Build history of the part. All positions in model axes, mm. Face numbers are marked on the shaded views. A direction names the side the tool comes from. Give positions to 0.01 mm unless a question says otherwise; leave off trailing zeros. Order: outer loops, then holes, each group sorted by start corner. A loop starts at its lowest first (then second) coordinate and runs counter-clockwise, first axis right, second up. Notation, with made-up numbers: (75, 83.25) - (96, 83.25) arc R21 ccw to (96, 122.25) - close; hole circle Ø1 at (43.5, -10.5). An arc over 180 degrees is marked (long way). Use a Markdown table: item, result.
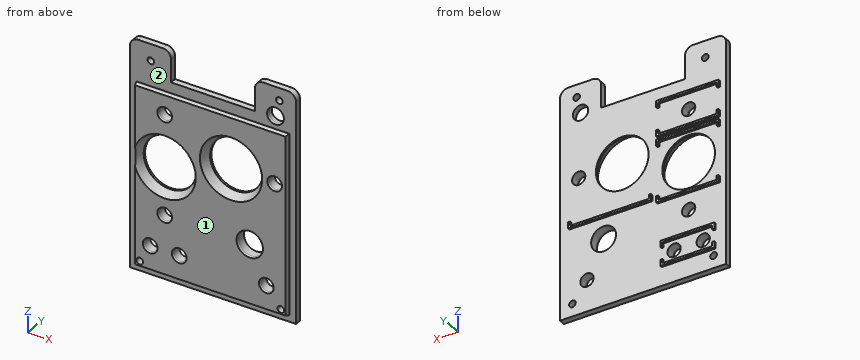
from build123d import *
from OCP.BRepFilletAPI import BRepFilletAPI_MakeChamfer

# Parameters (mm, degrees)
SKETCH1_W           = 80
SKETCH1_H           = 110
BOSS_EXTRUDE1_DEPTH = 3
SKETCH2_W           = 40.4
SKETCH2_H           = 3
CUT_EXTRUDE1_DEPTH  = 15
FILLET1_R           = 4
SKETCH7_W           = 73.6
SKETCH7_H           = 86.6
BOSS_EXTRUDE2_DEPTH = 2
SKETCH3_R           = 12.7
CUT_EXTRUDE2_DEPTH  = 69.190908485
SKETCH4_R           = 6
SKETCH4_R_2         = 3.2
SKETCH4_R_3         = 3.7
SKETCH4_R_4         = 1.6
CUT_EXTRUDE3_DEPTH  = 69.190908485
CHAMFER2_SIZE       = 1.5
CHAMFER2_SIZE2      = 0.545955351
CHAMFER3_SIZE       = 2.309401077
CHAMFER3_SIZE_2     = 4
BOSS_EXTRUDE3_DEPTH = 1
CHAMFER4_SIZE       = 1
CHAMFER4_SIZE2      = 0.363970234


with BuildPart() as part:
    # Sketch1 → Boss-Extrude1 (new body)
    with BuildSketch(Plane(origin=(0, 0, 0), x_dir=(1, 0, 0), z_dir=(0, 1, 0))):
        Rectangle(SKETCH1_W, SKETCH1_H)
    extrude(amount=BOSS_EXTRUDE1_DEPTH)

    # Sketch2 → Cut-Extrude1 (cut)
    with BuildSketch(Plane.XY.offset(55)):
        with Locations((0, 1.5)):
            Rectangle(SKETCH2_W, SKETCH2_H)
    extrude(amount=-CUT_EXTRUDE1_DEPTH, mode=Mode.SUBTRACT)

    # Fillet1
    fillet1_edges = [part.edges().sort_by_distance(p)[0] for p in [
        (-20.2, 1.5, 55),
        (20.2, 1.5, 55),
        (40, 1.5, 55),
        (-40, 1.5, 55),
    ]]
    fillet(fillet1_edges, radius=FILLET1_R)

    # Sketch7 → Boss-Extrude2 (add)
    with BuildSketch(Plane.XZ):
        with Locations((0, -8.5)):
            Rectangle(SKETCH7_W, SKETCH7_H)
    extrude(amount=BOSS_EXTRUDE2_DEPTH)

    # Sketch3 → Cut-Extrude2 (cut, through all)
    with BuildSketch(Plane(origin=(0, 3, 0), x_dir=(1, 0, 0), z_dir=(0, 1, 0))):
        with Locations(Location((-22, 0, 0), (0, 0, 270))):
            Circle(SKETCH3_R)
        with Locations(Location((10, -10, 0), (0, 0, 270))):
            Circle(SKETCH3_R)
    extrude(amount=-CUT_EXTRUDE2_DEPTH, mode=Mode.SUBTRACT)

    # Sketch4 → Cut-Extrude3 (cut, through all)
    with BuildSketch(Plane(origin=(0, 3, 0), x_dir=(1, 0, 0), z_dir=(0, 1, 0))):
        with Locations(Location((19, 23, 0), (0, 0, 270))):
            Circle(SKETCH4_R)
        with Locations(Location((-22, 23, 0), (0, 0, 270))):
            Circle(SKETCH4_R_2)
        with Locations(Location((31, -10, 0), (0, 0, 270))):
            Circle(SKETCH4_R_2)
        with Locations(Location((30.1, -41, 0), (0, 0, 270))):
            Circle(SKETCH4_R_3)
        with Locations(Location((-29, 40, 0), (0, 0, 270))):
            Circle(SKETCH4_R_2)
        with Locations(Location((-15, 40, 0), (0, 0, 270))):
            Circle(SKETCH4_R_2)
        with Locations(Location((27, 40, 0), (0, 0, 270))):
            Circle(SKETCH4_R_2)
        with Locations(Location((-22, -25, 0), (0, 0, 270))):
            Circle(SKETCH4_R_2)
        with Locations(Location((-30, -47, 0), (0, 0, 270))):
            Circle(SKETCH4_R_4)
        with Locations(Location((-34, 49, 0), (0, 0, 270))):
            Circle(SKETCH4_R_4)
        with Locations(Location((34, 49, 0), (0, 0, 270))):
            Circle(SKETCH4_R_4)
        with Locations(Location((32, -49, 0), (0, 0, 270))):
            Circle(SKETCH4_R_4)
    extrude(amount=-CUT_EXTRUDE3_DEPTH, mode=Mode.SUBTRACT)

    # Chamfer2: one chamfer whose edges measure the first distance from different faces: ONE call of the kernel's chamfer builder (chamfer() names one face for all edges)
    chamfer2_edges_1 = [part.edges().sort_by_distance(p)[0] for p in [
        (-36.8, -2, -8.5),
    ]]
    chamfer2_side_1 = [part.faces().sort_by_distance(p)[0] for p in [
        (-36.8, -1, -8.5),
    ]]
    chamfer2_edges_2 = [part.edges().sort_by_distance(p)[0] for p in [
        (0, -2, -51.8),
    ]]
    chamfer2_side_2 = [part.faces().sort_by_distance(p)[0] for p in [
        (0, -1, -51.8),
    ]]
    chamfer2_edges_3 = [part.edges().sort_by_distance(p)[0] for p in [
        (36.8, -2, -8.5),
    ]]
    chamfer2_side_3 = [part.faces().sort_by_distance(p)[0] for p in [
        (36.8, -1, -8.5),
    ]]
    chamfer2_edges_4 = [part.edges().sort_by_distance(p)[0] for p in [
        (0, -2, 34.8),
    ]]
    chamfer2_side_4 = [part.faces().sort_by_distance(p)[0] for p in [
        (0, -1, 34.8),
    ]]
    chamfer2 = BRepFilletAPI_MakeChamfer(part.part.solid().wrapped)
    for e in chamfer2_edges_1:
        chamfer2.Add(CHAMFER2_SIZE, CHAMFER2_SIZE2, e.wrapped, chamfer2_side_1[0].wrapped)  # the first distance lies on this face
    for e in chamfer2_edges_2:
        chamfer2.Add(CHAMFER2_SIZE, CHAMFER2_SIZE2, e.wrapped, chamfer2_side_2[0].wrapped)  # the first distance lies on this face
    for e in chamfer2_edges_3:
        chamfer2.Add(CHAMFER2_SIZE, CHAMFER2_SIZE2, e.wrapped, chamfer2_side_3[0].wrapped)  # the first distance lies on this face
    for e in chamfer2_edges_4:
        chamfer2.Add(CHAMFER2_SIZE, CHAMFER2_SIZE2, e.wrapped, chamfer2_side_4[0].wrapped)  # the first distance lies on this face
    add(Compound.cast(chamfer2.Shape()), mode=Mode.REPLACE)

    # Chamfer3
    # the kernel refuses this chamfer: 4, 2.309401077 mm, written as the material it takes off along each edge
    with BuildSketch(Plane(origin=(-22, -2, 0), x_dir=(0, 0, 1), z_dir=(-1, 0, 0))) as chamfer3_piece_1:
        Polygon((12.7 + CHAMFER3_SIZE, 0), (12.7, CHAMFER3_SIZE_2), (12.7, 0), align=None)
    revolve(axis=Axis((-22, -2, 0), (0, 1, 0)), mode=Mode.SUBTRACT)
    with BuildSketch(Plane(origin=(10, -2, 10), x_dir=(0, 0, 1), z_dir=(-1, 0, 0))) as chamfer3_piece_2:
        Polygon((12.7 + CHAMFER3_SIZE, 0), (12.7, CHAMFER3_SIZE_2), (12.7, 0), align=None)
    revolve(axis=Axis((10, -2, 10), (0, 1, 0)), mode=Mode.SUBTRACT)

    # Sketch8 → Boss-Extrude3 (add)
    with BuildSketch(Plane(origin=(0, 3, 0), x_dir=(1, 0, 0), z_dir=(0, 1, 0))):
        Polygon((-35, 43), (-35, 46), (-9, 46), (-9, 43), (-10, 43), (-10, 45), (-34, 45), (-34, 43), align=None)
        Polygon((-9, 37), (-9, 34), (-35, 34), (-35, 37), (-34, 37), (-34, 35), (-10, 35), (-10, 37), align=None)
        Polygon((-37, 12), (-37, 15), (-7, 15), (-7, 12), (-8, 12), (-8, 14), (-36, 14), (-36, 12), align=None)
        Polygon((-4.5, 10), (-4.5, 13), (35.5, 13), (35.5, 10), (34.5, 10), (34.5, 12), (-3.5, 12), (-3.5, 10), align=None)
        Polygon((-7, -12), (-7, -15), (-37, -15), (-37, -12), (-36, -12), (-36, -14), (-8, -14), (-8, -12), align=None)
        Polygon((-37, -19.5), (-37, -16.5), (-7, -16.5), (-7, -19.5), (-8, -19.5), (-8, -17.5), (-36, -17.5), (-36, -19.5), align=None)
        Polygon((-7, -30.5), (-7, -33.5), (-37, -33.5), (-37, -30.5), (-36, -30.5), (-36, -32.5), (-8, -32.5), (-8, -30.5), align=None)
    extrude(amount=BOSS_EXTRUDE3_DEPTH)

    # Chamfer4: one chamfer whose edges measure the first distance from different faces: ONE call of the kernel's chamfer builder (chamfer() names one face for all edges)
    chamfer4_edges_1 = [part.edges().sort_by_distance(p)[0] for p in [
        (-22, -2, 21.8),
    ]]
    chamfer4_side_1 = [part.faces().sort_by_distance(p)[0] for p in [
        (-22, 0.5, 21.8),
    ]]
    chamfer4_edges_2 = [part.edges().sort_by_distance(p)[0] for p in [
        (-22, -2, -26.2),
    ]]
    chamfer4_side_2 = [part.faces().sort_by_distance(p)[0] for p in [
        (-22, 0.5, -26.2),
    ]]
    chamfer4_edges_3 = [part.edges().sort_by_distance(p)[0] for p in [
        (31, -2, 6.8),
    ]]
    chamfer4_side_3 = [part.faces().sort_by_distance(p)[0] for p in [
        (31, 0.5, 6.8),
    ]]
    chamfer4_edges_4 = [part.edges().sort_by_distance(p)[0] for p in [
        (30.1, 0, 37.3),
    ]]
    chamfer4_side_4 = [part.faces().sort_by_distance(p)[0] for p in [
        (30.1, 1.5, 37.3),
    ]]
    chamfer4_edges_5 = [part.edges().sort_by_distance(p)[0] for p in [
        (-29, -2, -43.2),
    ]]
    chamfer4_side_5 = [part.faces().sort_by_distance(p)[0] for p in [
        (-29, 0.5, -43.2),
    ]]
    chamfer4_edges_6 = [part.edges().sort_by_distance(p)[0] for p in [
        (-15, -2, -43.2),
    ]]
    chamfer4_side_6 = [part.faces().sort_by_distance(p)[0] for p in [
        (-15, 0.5, -43.2),
    ]]
    chamfer4_edges_7 = [part.edges().sort_by_distance(p)[0] for p in [
        (19, -2, -29),
    ]]
    chamfer4_side_7 = [part.faces().sort_by_distance(p)[0] for p in [
        (19, 0.5, -29),
    ]]
    chamfer4_edges_8 = [part.edges().sort_by_distance(p)[0] for p in [
        (27, -2, -43.2),
    ]]
    chamfer4_side_8 = [part.faces().sort_by_distance(p)[0] for p in [
        (27, 0.5, -43.2),
    ]]
    chamfer4 = BRepFilletAPI_MakeChamfer(part.part.solid().wrapped)
    for e in chamfer4_edges_1:
        chamfer4.Add(CHAMFER4_SIZE, CHAMFER4_SIZE2, e.wrapped, chamfer4_side_1[0].wrapped)  # the first distance lies on this face
    for e in chamfer4_edges_2:
        chamfer4.Add(CHAMFER4_SIZE, CHAMFER4_SIZE2, e.wrapped, chamfer4_side_2[0].wrapped)  # the first distance lies on this face
    for e in chamfer4_edges_3:
        chamfer4.Add(CHAMFER4_SIZE, CHAMFER4_SIZE2, e.wrapped, chamfer4_side_3[0].wrapped)  # the first distance lies on this face
    for e in chamfer4_edges_4:
        chamfer4.Add(CHAMFER4_SIZE, CHAMFER4_SIZE2, e.wrapped, chamfer4_side_4[0].wrapped)  # the first distance lies on this face
    for e in chamfer4_edges_5:
        chamfer4.Add(CHAMFER4_SIZE, CHAMFER4_SIZE2, e.wrapped, chamfer4_side_5[0].wrapped)  # the first distance lies on this face
    for e in chamfer4_edges_6:
        chamfer4.Add(CHAMFER4_SIZE, CHAMFER4_SIZE2, e.wrapped, chamfer4_side_6[0].wrapped)  # the first distance lies on this face
    for e in chamfer4_edges_7:
        chamfer4.Add(CHAMFER4_SIZE, CHAMFER4_SIZE2, e.wrapped, chamfer4_side_7[0].wrapped)  # the first distance lies on this face
    for e in chamfer4_edges_8:
        chamfer4.Add(CHAMFER4_SIZE, CHAMFER4_SIZE2, e.wrapped, chamfer4_side_8[0].wrapped)  # the first distance lies on this face
    add(Compound.cast(chamfer4.Shape()), mode=Mode.REPLACE)


solid = part.part
1) Pin check, flat tips, straight feed: P1, Ø0.5, axis at y = 3.5, z = 13.5, coming from the -X side; P2, Ø0.5, axis at y = 3.5, z = -11.5, coming from the -X side; P3, Ø1.1, axis at x = -23.5, y = 3.5, coming from the +Z side. Stop position of each tip, or through.
Computed:
| item | result |
|---|---|
| P1 | stops at x = -37 |
| P2 | stops at x = -4.5 |
| P3 | stops at z = 54.97 |
2) Slice it at A-A (z = -40). Write the cut outline in (x, y), and give its area (3 significant figures).
Computed:
| item | result |
|---|---|
| outline | (-40, 0) - (-36.8, 0) - (-36.8, -0.5) - (-36.25, -2) - (-32.56, -2) - (-32.2, -1) - (-32.2, 3) - (-40, 3) - close; (-25.8, -1) - (-25.44, -2) - (-18.56, -2) - (-18.2, -1) - (-18.2, 3) - (-25.8, 3) - close; (-11.8, -1) - (-11.44, -2) - (23.44, -2) - (23.8, -1) - (23.8, 3) - (-11.8, 3) - close; (30.2, -1) - (30.56, -2) - (36.25, -2) - (36.8, -0.5) - (36.8, 0) - (40, 0) - (40, 3) - (30.2, 3) - close |
| area | 289 mm² |
3) Slice it at B-B (x = 19). State how many separate pieces and enclosed holes the cut face has, and give its area (3 significant figures).
Computed:
| item | result |
|---|---|
| separate pieces | 3 |
| enclosed holes | 0 |
| area | 296 mm² |
4) Tool access for the marked faces 1 and 2: list every direction of +Z, -Z, +X, -X, +Y, -Y with a clear straight run to the whole face (end or side of a thin tool).
Computed:
| item | result |
|---|---|
| face 1 | +Z, -Z, +X, -X, -Y |
| face 2 | -Y |
5) Wall check: line 1 (X direction, y = 1.7, z = 47); line 2 (X direction, y = 2.1, z = 25); line 3 (X direction, y = 1.2, z = -23). Give the ranges that are in metal, low to high. Write a range as from..to.
Computed:
| item | result |
|---|---|
| line 1 | x = -40..-31.6, -28.4..-20.2, 20.2..40 |
| line 2 | x = -40..-25.2, -18.8..40 |
| line 3 | x = -40..-25.2, -18.8..13, 25..40 |
